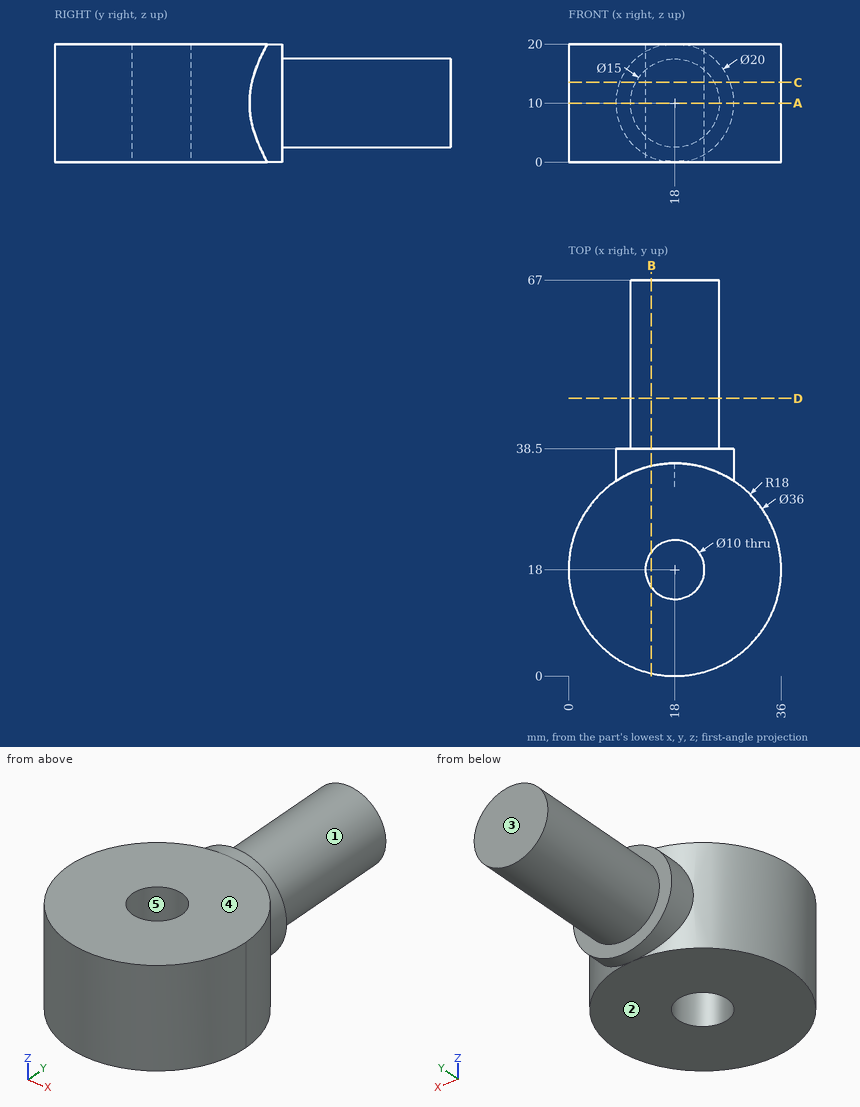
The figure shows three views and two pictorial views of one solid part (mm, origin at its lowest corner). Answer the questions. A direction names the side the tool comes from. Give positions to 0.01 mm unless a question says otherwise; leave off trailing zeros. Order: outer loops, then holes, each group sorted by start corner. A loop starts at its lowest first (then second) coordinate and runs counter-clockwise, first axis right, second up. Notation, with made-up numbers: (17, 6.5) -> (56, 6.5) arc R25 cw to (56, 42.5) -> close; hole circle Ø7 at (42.5, 75). An arc over 180 degrees is marked (long way). Answer as CSV lines item,"result". Start each with the question number.
Q1. A cutting plane is placed at B-B (x = 14). Determine the outline of the cut face in (y, z), then the cut area to 3 significant figures.
Q2. Find the intervals of material crossed by L1, parallel to Y at x = 18, z = 10; L2, parallel to X at y = 60.5, z = 10; L3, parallel to X at y = 18.5, z = 17.75, in increasing order.
Q3. A cutting plane is placed at C-C (z = 13.5). Determine the outline of the cut face in (x, y), then the cut area to 3 significant figures.
Q4. Determine the mould class of the marked faces 3, 4 and 5 for opening direction Y: pulls with the +Y half, pulls with the -Y half, needs draft (parallel to the pull), parting line crosses it, or undercut.
Q5. Given pin 1 (6 mm diameter, centred on x = 15, z = 8.5, fed in from -Y); pin 2 (1 mm diameter, centred on x = 24.5, z = 3.5, fed in from +Y); pin 3 (4 mm diameter, centred on x = 5, z = 17, fed in from +Y); pin 4 (12 mm diameter, centred on x = 7.5, z = 18, fed in from -Y), each flat-ended and moving along its own axis, determine where each tip first touches the part or whether it passes through.
Q6. A cutting plane is placed at D-D (y = 47). Determine the outline of the cut face in (x, z), then the cut area to 3 significant figures.
Q7. Which of the six approach directions +Z, -Z, +X, -X, +Y, -Y give full straight-line access (tool end or side, diameter ignored) to the marked faces 1 and 2?
Q8. A cutting plane is placed at A-A (z = 10). Determine the outline of the cut face in (x, y), then the cut area to 3 significant figures.
Results found:
1,outline,"(0.45, 0) -> (15, 0) -> (15, 20) -> (0.45, 20) -> close; (21, 0) -> (35.55, 0) -> (35.55, 0.83) -> (38.5, 0.83) -> (38.5, 3.66) -> (67, 3.66) -> (67, 16.34) -> (38.5, 16.34) -> (38.5, 19.17) -> (35.55, 19.17) -> (35.55, 20) -> (21, 20) -> close"
1,area,"998 mm2"
2,L1,"0 to 13, 23 to 67"
2,L2,"10.5 to 25.5"
2,L3,"0.01 to 13.03, 22.97 to 35.99"
3,outline,"(8.63, 33.37) arc R18 ccw (long way) to (27.37, 33.37) -> (27.37, 38.5) -> (24.63, 38.5) -> (24.63, 67) -> (11.37, 67) -> (11.37, 38.5) -> (8.63, 38.5) -> close; hole circle Ø10 at (18, 18)"
3,area,"1,380 mm2"
4,face 3,"pulls with the +Y half"
4,face 4,"needs draft"
4,face 5,"undercut"
5,pin 1,"y = 0"
5,pin 2,"y = 38.5"
5,pin 3,"y = 32.25"
5,pin 4,"y = 0.57"
6,outline,"circle Ø15 at (18, 10)"
6,area,"177 mm2"
7,face 1,"+Y"
7,face 2,"-Z, +X, -X, +Y, -Y"
8,outline,"(8, 32.97) arc R18 ccw (long way) to (28, 32.97) -> (28, 38.5) -> (25.5, 38.5) -> (25.5, 67) -> (10.5, 67) -> (10.5, 38.5) -> (8, 38.5) -> close; hole circle Ø10 at (18, 18)"
8,area,"1,440 mm2"
